Source: three-view drawing plus pictorial views. Frame: mm from the lowest corner of the part. Round coordinates to 2 decimals unless told otherwise and drop trailing zeros. Order: outer loops, then holes, each group sorted by start corner. A loop starts at its lowest first (then second) coordinate and runs counter-clockwise, first axis right, second up. Notation, with made-up numbers: (86, 33) -> (113, 33) arc R20 ccw to (113, 47) -> close; hole circle Ø10 at (17.5, 1). An arc over 180 degrees is marked (long way). Answer as CSV lines item,"result".
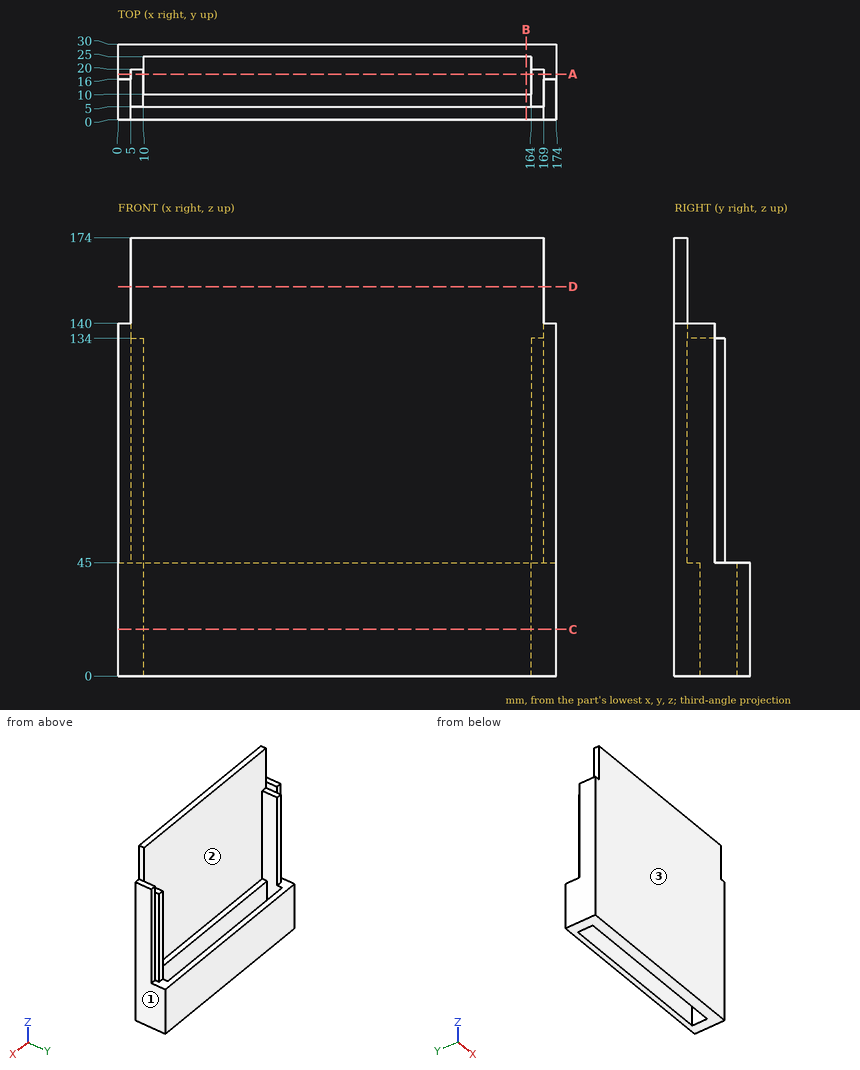
1. Line query: L1, parallel to Y at x = 31.5, z = 22; L2, parallel to X at y = 15, z = 68; L3, parallel to X at y = 16.5, z = 62. Output: solid intervals per line, ascending. Write a range as [from, to].
Results below:
L1,"[0, 10], [25, 30]"
L2,"[0, 10], [164, 174]"
L3,"[5, 10], [164, 169]"
2. Pin query (flat end, axial travel): pin 1 (1.5 mm diameter, centred on x = 115.5, y = 10.5, fed in from -Z); pin 2 (5.5 mm diameter, centred on x = 167, y = 9, fed in from +Z); pin 3 (1.5 mm diameter, centred on x = 8.5, y = 12.5, fed in from +Z); pin 4 (4 mm diameter, centred on x = 1.5, z = 92, fed in from +Y). Return the tip coordinate at first contact, or that it passes through.
Results below:
pin 1,"z = 0"
pin 2,"z = 140"
pin 3,"z = 134"
pin 4,"y = 16"
3. Section query B-B on x = 162. Return loops of the section in (y, z), and give its area (3 significant figures).
Results below:
outline,"(0, 0) -> (10, 0) -> (10, 45) -> (5, 45) -> (5, 174) -> (0, 174) -> close; (25, 0) -> (30, 0) -> (30, 45) -> (25, 45) -> close"
area,"1,320 mm2"
4. Section query A-A on y = 18. Return loops of the section in (x, z), and give its area (3 significant figures).
Results below:
outline,"(0, 0) -> (10, 0) -> (10, 134) -> (5, 134) -> (5, 45) -> (0, 45) -> close; (164, 0) -> (174, 0) -> (174, 45) -> (169, 45) -> (169, 134) -> (164, 134) -> close"
area,"1,790 mm2"
5. Section query D-D on z = 154.5. Return loops of the section in (x, y), and give its area (3 significant figures).
Results below:
outline,"(5, 0) -> (169, 0) -> (169, 5) -> (5, 5) -> close"
area,"820 mm2"
6. Section query C-C on z = 18.5. Return loops of the section in (x, y), and give its area (3 significant figures).
Results below:
outline,"(0, 0) -> (174, 0) -> (174, 30) -> (0, 30) -> close; hole (10, 10) -> (164, 10) -> (164, 25) -> (10, 25) -> close"
area,"2,910 mm2"
7. Mould query, pull axis X, two halves, no side actions, for the marked faces 1, 2 and 3. Classes: released by +X, released by -X, zero draft, split by the parting line, or undercut.
Results below:
face 1,"released by +X"
face 2,"undercut"
face 3,"zero draft"
